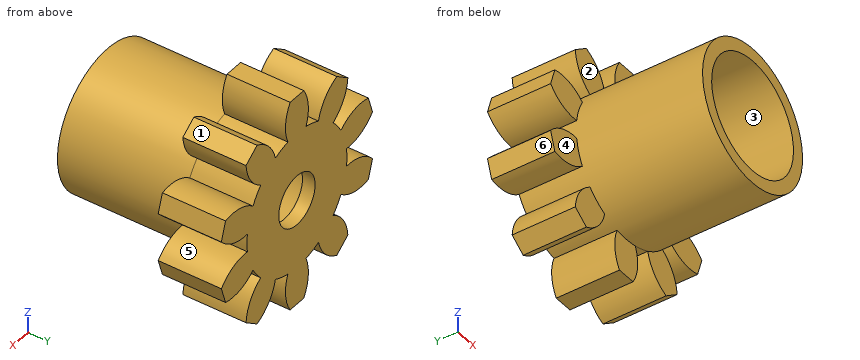
from build123d import *
from build123d.topology import SkipClean

# Parameters (mm, degrees)
SKETCH_1_R      = 5.5
EXTRUDE_1_DEPTH = 5
EXTRUDE_START   = -5
EXTRUDE_2_DEPTH = 5
EXTRUDE_START_2 = 10
SKETCH_3_R      = 5.5
EXTRUDE_3_DEPTH = 10


with BuildPart() as part:
    # 草图1 → 凸台-拉伸1 (new body)
    with BuildSketch(Plane(origin=(0, 0, 0), x_dir=(1, 0, 0), z_dir=(0, 1, 0))):
        with Locations(Location((0, 0, 0), (0, 0, 270))):
            Circle(SKETCH_1_R)
    extrude(amount=EXTRUDE_1_DEPTH)

    # 草图2 → 凸台-拉伸2 (add)
    with BuildSketch(Plane(origin=(0, 5, 0), x_dir=(-1, 0, 0), z_dir=(0, 1, 0)).offset(EXTRUDE_START)):
        with BuildLine():
            Line((-4.389411899, -7.317483391), (-5.60293739, -6.435805513))
            ThreePointArc((-5.60293739, -6.435805513), (-5.11774735, -4.915167527), (-3.987951794, -3.787643132))
            ThreePointArc((-3.987951794, -3.787643132), (-3.232818888, -4.449593469), (-2.369917805, -4.963213636))
            ThreePointArc((-2.369917805, -4.963213636), (-3.093131201, -6.386137262), (-4.389411899, -7.317483391))
        make_face()
        with BuildLine():
            Line((-7.852217643, -3.339936839), (-8.315743134, -1.913352065))
            ThreePointArc((-8.315743134, -1.913352065), (-7.029407564, -0.968317642), (-5.452641547, -0.720208411))
            ThreePointArc((-5.452641547, -0.720208411), (-5.23081084, -1.699593469), (-4.834607559, -2.622321444))
            ThreePointArc((-4.834607559, -2.622321444), (-6.256073009, -3.34839667), (-7.852217643, -3.339936839))
        make_face()
        with BuildLine():
            Line((-8.315743134, 1.913352065), (-7.852217643, 3.339936839))
            ThreePointArc((-7.852217643, 3.339936839), (-6.256073009, 3.34839667), (-4.834607559, 2.622321444))
            ThreePointArc((-4.834607559, 2.622321444), (-5.23081084, 1.699593469), (-5.452641547, 0.720208411))
            ThreePointArc((-5.452641547, 0.720208411), (-7.029407564, 0.968317642), (-8.315743134, 1.913352065))
        make_face()
        with BuildLine():
            Line((-5.60293739, 6.435805513), (-4.389411899, 7.317483391))
            ThreePointArc((-4.389411899, 7.317483391), (-3.093131201, 6.386137262), (-2.369917805, 4.963213636))
            ThreePointArc((-2.369917805, 4.963213636), (-3.232818888, 4.449593469), (-3.987951794, 3.787643132))
            ThreePointArc((-3.987951794, 3.787643132), (-5.11774735, 4.915167527), (-5.60293739, 6.435805513))
        make_face()
        with BuildLine():
            Line((-0.75, 8.5), (0.75, 8.5))
            ThreePointArc((0.75, 8.5), (1.251281594, 6.984590476), (1, 5.408326913))
            ThreePointArc((1, 5.408326913), (0, 5.5), (-1, 5.408326913))
            ThreePointArc((-1, 5.408326913), (-1.251281594, 6.984590476), (-0.75, 8.5))
        make_face()
        with BuildLine():
            Line((4.389411899, 7.317483391), (5.60293739, 6.435805513))
            ThreePointArc((5.60293739, 6.435805513), (5.11774735, 4.915167527), (3.987951794, 3.787643132))
            ThreePointArc((3.987951794, 3.787643132), (3.232818888, 4.449593469), (2.369917805, 4.963213636))
            ThreePointArc((2.369917805, 4.963213636), (3.093131201, 6.386137262), (4.389411899, 7.317483391))
        make_face()
        with BuildLine():
            Line((0.75, -8.5), (-0.75, -8.5))
            ThreePointArc((-0.75, -8.5), (-1.251281594, -6.984590476), (-1, -5.408326913))
            ThreePointArc((-1, -5.408326913), (0, -5.5), (1, -5.408326913))
            ThreePointArc((1, -5.408326913), (1.251281594, -6.984590476), (0.75, -8.5))
        make_face()
        with BuildLine():
            Line((7.852217643, 3.339936839), (8.315743134, 1.913352065))
            ThreePointArc((8.315743134, 1.913352065), (7.029407564, 0.968317642), (5.452641547, 0.720208411))
            ThreePointArc((5.452641547, 0.720208411), (5.23081084, 1.699593469), (4.834607559, 2.622321444))
            ThreePointArc((4.834607559, 2.622321444), (6.256073009, 3.34839667), (7.852217643, 3.339936839))
        make_face()
        with BuildLine():
            Line((8.315743134, -1.913352065), (7.852217643, -3.339936839))
            ThreePointArc((7.852217643, -3.339936839), (6.256073009, -3.34839667), (4.834607559, -2.622321444))
            ThreePointArc((4.834607559, -2.622321444), (5.23081084, -1.699593469), (5.452641547, -0.720208411))
            ThreePointArc((5.452641547, -0.720208411), (7.029407564, -0.968317642), (8.315743134, -1.913352065))
        make_face()
        with BuildLine():
            Line((5.60293739, -6.435805513), (4.389411899, -7.317483391))
            ThreePointArc((4.389411899, -7.317483391), (3.093131201, -6.386137262), (2.369917805, -4.963213636))
            ThreePointArc((2.369917805, -4.963213636), (3.232818888, -4.449593469), (3.987951794, -3.787643132))
            ThreePointArc((3.987951794, -3.787643132), (5.11774735, -4.915167527), (5.60293739, -6.435805513))
        make_face()
    extrude(amount=EXTRUDE_2_DEPTH)

    # 草图3 → 凸台-拉伸3 (add)
    with SkipClean():  # the faces are left unmerged after this step: merging them gives an invalid solid
        with BuildSketch(Plane.XZ.offset(EXTRUDE_START_2)):
            with Locations(Location((0, 0, 0), (0, 0, 270))):
                Circle(SKETCH_3_R)
        extrude(amount=-EXTRUDE_3_DEPTH)

    # 草图4 → 切除-旋转1 (revolve, cut)
    with SkipClean():  # the faces are left unmerged after this step: merging them gives an invalid solid
        with BuildSketch(Plane.XY, mode=Mode.PRIVATE) as cut_revolve_1_sk:
            Polygon((0, -10), (0, -3), (0, 4), (0, 5), (2, 5), (2, 4), (3, 4), (4.5, -3), (4.5, -10), align=None)
        revolve(cut_revolve_1_sk.sketch.rotate(Axis((0, -3, 0), (0, 1, 0)), 90), axis=Axis((0, -3, 0), (0, 1, 0)), mode=Mode.SUBTRACT)


solid = part.part
Check sheet for the modelled part. Datum: model origin and axes. Units: mm. Face numbers are marked on the shaded views. A direction names the side the tool comes from. Round coordinates to 2 decimals unless told otherwise and drop trailing zeros. Loops run counter-clockwise (first coordinate to the right, second up) from the corner with the lowest first, then second, coordinate; pieces in that order, holes last. Notation, with made-up numbers: M -27,69 L 21,69 A28 ccw 21,100 Z; hole C 57,19.5 d11. An arc over 180 degrees is marked long. One line per question, with ' | ' between items. Start each with the question number.
Item 1: Scan lines: probe 1 along X at (y, z) = (4.5, 0); probe 2 along X at (y, z) = (-4.25, 0); probe 3 along Y at (x, z) = (-4.5, -6). Record each from-to range of solid material in increasing order.
Item 2: Set-up check for the marked faces 1, 2 and 3: record each of +Z, -Z, +X, -X, +Y, -Y from which the full face is reachable in a straight line by a thin tool's end or side.
Item 3: Section check C-C (y = -4.75). Record the boundary of the cut face in (x, z), and give its area (3 significant figures).
Item 4: Section check A-A (z = 0). Record the boundary of the cut face in (x, y), and give its area (3 significant figures).
Item 5: Gauge pin test, flat ends, axial feed: pin 1 Ø1 at (x, z) = (3.5, -5) entering from -Y; pin 2 Ø4.5 at (x, z) = (0, 0) entering from -Y. Record the tip position at first contact, or that the pin passes through.
Item 6: Section check D-D (x = -6). Record the boundary of the cut face in (y, z).
Item 7: Section check B-B (x = 0). Record the boundary of the cut face in (y, z).
Item 8: Release check for a two-part mould opening along Z. For the marked faces 4, 5 and 6 record: released by +Z, released by -Z, zero draft, split by the parting line, or undercut.
Worked out:
1) probe 1: -5.5 to -2, 2 to 5.5 | probe 2: -5.5 to -4.5, 4.5 to 5.5 | probe 3: 0 to 5
2) face 1: +Z, +X, +Y, -Y | face 2: +Z, -X, -Y | face 3: -Y
3) outline: C 0,0 d11; hole C 0,0 d9 | area: 31.4 mm^2
4) outline: M -5.5,-10 L -4.5,-10 L -4.5,-3 L -3,4 L -2,4 L -2,5 L -5.5,5 Z; M 2,4 L 3,4 L 4.5,-3 L 4.5,-10 L 5.5,-10 L 5.5,5 L 2,5 Z | area: 45.5 mm^2
5) pin 1: y = 0 | pin 2: y = 4
6) outline: M 0,-3.28 L 5,-3.28 L 5,-0.72 L 0,-0.72 Z; M 0,0.72 L 5,0.72 L 5,3.28 L 0,3.28 Z
7) outline: M -10,-5.5 L 0,-5.5 L 0,-8.5 L 5,-8.5 L 5,-2 L 4,-2 L 4,-3 L -3,-4.5 L -10,-4.5 Z; M -10,4.5 L -3,4.5 L 4,3 L 4,2 L 5,2 L 5,8.5 L 0,8.5 L 0,5.5 L -10,5.5 Z
8) face 4: zero draft | face 5: undercut | face 6: released by -Z
